Here's how the part is built. I have some questions about the finished solid (model axes, mm). Face numbers are marked on the shaded views. Coordinates: 2 decimals unless noted, no trailing zeros. Write each loop counter-clockwise with the first axis right and the second up, starting at its lowest first coordinate (ties: lowest second). Pieces come first, ordered by that corner, then holes. Notation, with made-up numbers: M -1,83 L 42,83 A6 cw 42,92 Z; hole C 5.25,23 d6. An arc over 180 degrees is marked long. Use a Markdown table: item, result.
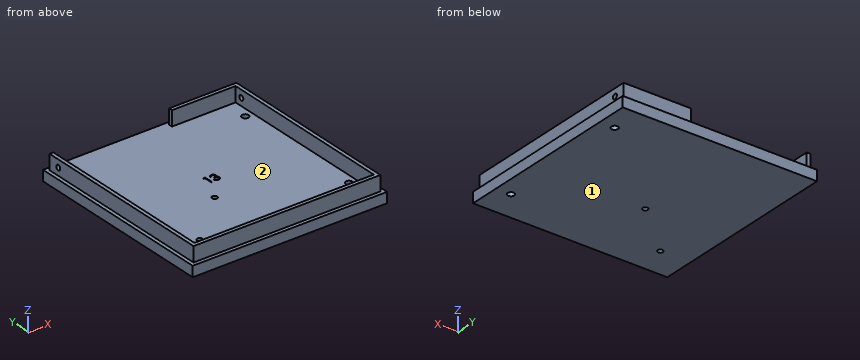
```python
from build123d import *

# Parameters (mm, degrees)
CROQUIS1_W              = 130
CROQUIS1_H              = 130
CROQUIS1_R              = 1.75
CROQUIS1_R_2            = 2.25
SALIENTE_EXTRUIR1_DEPTH = 7
CORTAR_EXTRUIR1_DEPTH   = 2
CROQUIS4_W              = 125
CROQUIS4_H              = 125
CROQUIS4_W_2            = 120
CROQUIS4_H_2            = 120
SALIENTE_EXTRUIR2_DEPTH = 10
CROQUIS6_R              = 1.7
CORTAR_EXTRUIR2_DEPTH   = 145.118874545
CORTAR_EXTRUIR3_REACH   = 146.119
CROQUIS7_W              = 77.5
CROQUIS7_H              = 10


with BuildPart() as part:
    # Croquis1 → Saliente-Extruir1 (new body)
    with BuildSketch(Plane.XY):
        Rectangle(CROQUIS1_W, CROQUIS1_H)
        with Locations((-11, -14)):
            Circle(CROQUIS1_R, mode=Mode.SUBTRACT)
        with Locations((-45, -45)):
            Circle(CROQUIS1_R, mode=Mode.SUBTRACT)
        with Locations((55, 45)):
            Circle(CROQUIS1_R_2, mode=Mode.SUBTRACT)
        with Locations((55, -45)):
            Circle(CROQUIS1_R_2, mode=Mode.SUBTRACT)
    extrude(amount=SALIENTE_EXTRUIR1_DEPTH)

    # Croquis2 → Cortar-Extruir1 (cut)
    with BuildSketch(Plane.XY.offset(7)):
        Polygon((-3.109375, 6), (-2, 6), (-2, 0), (-2.538461538, 0), (-2.538461538, 5.384615385), (-3.461538462, 5.384615385), align=None)
        with BuildLine():
            Line((1, 4.615384615), (0.461538462, 4.615384615))
            add(Edge.make_bspline(
                [(0.461538462, 4.615384615), (0.476126263, 4.675783159), (0.504644221, 4.793857373), (0.564125775, 4.962555534), (0.628924499, 5.122195856), (0.706734392, 5.269789126), (0.791606542, 5.40830153), (0.888845493, 5.534591458), (0.993965018, 5.651870827), (1.110236359, 5.755950663), (1.232171208, 5.850198199), (1.361487699, 5.93055544), (1.495584088, 5.999682559), (1.635389459, 6.056631528), (1.781320039, 6.099532426), (1.932056536, 6.130658378), (2.087993965, 6.150871717), (2.193846977, 6.152844454), (2.247596154, 6.153846154)],
                knots=[0, 0, 0, 0, 1.162005537, 2.271625781, 3.343758855, 4.383309926, 5.390229558, 6.379919256, 7.361854164, 8.333198761, 9.295911338, 10.242430842, 11.177959212, 12.116337295, 13.062827104, 14.020064771, 14.994644689, 16, 16, 16, 16], degree=3))
            add(Edge.make_bspline(
                [(2.247596154, 6.153846154), (2.325909426, 6.151481759), (2.48082773, 6.146804544), (2.708421525, 6.104094082), (2.927896072, 6.03650814), (3.136849069, 5.943124608), (3.33093781, 5.827946357), (3.503628416, 5.690863951), (3.652580149, 5.534522291), (3.777541939, 5.361837895), (3.875384795, 5.177285593), (3.947532863, 4.987342467), (3.991455745, 4.792459087), (3.997148128, 4.66087518), (4, 4.594951923)],
                knots=[0, 0, 0, 0, 1.083050992, 2.142477498, 3.193116406, 4.255571735, 5.30263384, 6.308962982, 7.297363603, 8.282367274, 9.249857812, 10.179914175, 11.08814088, 12, 12, 12, 12], degree=3))
            add(Edge.make_bspline(
                [(4, 4.594951923), (3.998005272, 4.531511704), (3.9941019, 4.407369039), (3.960958405, 4.226132187), (3.905181954, 4.055318015), (3.827919504, 3.894207451), (3.727905418, 3.743822011), (3.606752223, 3.603823341), (3.463604803, 3.473590499), (3.355126624, 3.398985688), (3.299278846, 3.360576923)],
                knots=[0, 0, 0, 0, 1.024540389, 2.004866551, 2.965041327, 3.920577974, 4.882998113, 5.874504559, 6.905732034, 8, 8, 8, 8], degree=3))
            add(Edge.make_bspline(
                [(3.299278846, 3.360576923), (3.363104711, 3.3297572), (3.48956221, 3.268694416), (3.661934546, 3.148941689), (3.818410904, 3.010673665), (3.905674422, 2.902771974), (3.949519231, 2.848557692)],
                knots=[0, 0, 0, 0, 1.015518401, 2.012035669, 3.001164323, 4, 4, 4, 4], degree=3))
            add(Edge.make_bspline(
                [(3.949519231, 2.848557692), (3.978390103, 2.809030118), (4.035659068, 2.730622261), (4.106348554, 2.604559817), (4.170478465, 2.477100121), (4.220450269, 2.344826853), (4.259148327, 2.209273116), (4.286810096, 2.070206151), (4.303994338, 1.927512398), (4.306455284, 1.830976718), (4.307692308, 1.782451923)],
                knots=[0, 0, 0, 0, 1.025084078, 2.033381695, 3.024893161, 4.013698104, 4.991890475, 5.976764909, 6.982997093, 8, 8, 8, 8], degree=3))
            add(Edge.make_bspline(
                [(4.307692308, 1.782451923), (4.304615999, 1.698435258), (4.298477858, 1.530797312), (4.243613731, 1.283126361), (4.158562461, 1.0410255), (4.037779142, 0.809468632), (3.890577699, 0.592816551), (3.715450857, 0.39897145), (3.514388443, 0.232345271), (3.290150187, 0.093127737), (3.047206539, -0.01816013), (2.787362667, -0.09540146), (2.514362574, -0.145708888), (2.327150064, -0.151103521), (2.231971154, -0.153846154)],
                knots=[0, 0, 0, 0, 0.955779014, 1.907060117, 2.875433937, 3.871313158, 4.872415639, 5.851225146, 6.836215519, 7.83643374, 8.849228613, 9.86973379, 10.916971861, 12, 12, 12, 12], degree=3))
            add(Edge.make_bspline(
                [(2.231971154, -0.153846154), (2.167823782, -0.152357788), (2.041603145, -0.149429181), (1.856042862, -0.129408722), (1.678919949, -0.092842999), (1.509994924, -0.043637332), (1.349117718, 0.018748511), (1.196779252, 0.096437708), (1.052042292, 0.187828854), (0.916272662, 0.294000719), (0.789486545, 0.41276873), (0.675053304, 0.546241319), (0.571065087, 0.691951154), (0.480306278, 0.851590679), (0.398642931, 1.023096834), (0.331475577, 1.208665688), (0.272357459, 1.406638298), (0.24487152, 1.544600138), (0.230769231, 1.615384615)],
                knots=[0, 0, 0, 0, 1.048658725, 2.063410685, 3.046034179, 4.001477787, 4.936774919, 5.862367409, 6.792675028, 7.730719943, 8.675894397, 9.627829632, 10.600096036, 11.597688215, 12.626045268, 13.701542398, 14.82072376, 16, 16, 16, 16], degree=3))
            Line((0.230769231, 1.615384615), (0.769230769, 1.615384615))
            add(Edge.make_bspline(
                [(0.769230769, 1.615384615), (0.783259269, 1.569186307), (0.810545919, 1.479326584), (0.856993287, 1.350000346), (0.909910325, 1.231443683), (0.96667814, 1.122786903), (1.026298333, 1.022959927), (1.093009633, 0.934602437), (1.161871025, 0.853833519), (1.213778488, 0.80832847), (1.239182692, 0.786057692)],
                knots=[0, 0, 0, 0, 1.198163088, 2.33053128, 3.407730985, 4.417276592, 5.372219308, 6.28897303, 7.162600585, 8, 8, 8, 8], degree=3))
            add(Edge.make_bspline(
                [(1.239182692, 0.786057692), (1.272776823, 0.760157691), (1.339861388, 0.708437637), (1.449178356, 0.642434845), (1.564146732, 0.585244516), (1.687257602, 0.54155818), (1.815854352, 0.504567905), (1.952015549, 0.480361301), (2.094539921, 0.463753007), (2.191856087, 0.46228741), (2.241586538, 0.461538462)],
                knots=[0, 0, 0, 0, 0.946170439, 1.889420265, 2.845303464, 3.807233317, 4.801018734, 5.828864929, 6.890507805, 8, 8, 8, 8], degree=3))
            add(Edge.make_bspline(
                [(2.241586538, 0.461538462), (2.2977354, 0.462594299), (2.407529652, 0.464658898), (2.567737982, 0.483645824), (2.72015075, 0.511297962), (2.863075765, 0.554005932), (2.998385206, 0.606773106), (3.12418232, 0.673027515), (3.242118502, 0.750761324), (3.350683197, 0.839114167), (3.448304067, 0.93583673), (3.534257518, 1.037001995), (3.607328367, 1.142183417), (3.666271643, 1.251963053), (3.712815444, 1.365886303), (3.744500931, 1.484272867), (3.766532099, 1.606153895), (3.768326292, 1.689003556), (3.769230769, 1.730769231)],
                knots=[0, 0, 0, 0, 1.217147791, 2.380027433, 3.494444702, 4.572153297, 5.609568379, 6.639424714, 7.649109417, 8.668170816, 9.669597737, 10.625200337, 11.543417969, 12.441394052, 13.322311151, 14.205496177, 15.095365482, 16, 16, 16, 16], degree=3))
            add(Edge.make_bspline(
                [(3.769230769, 1.730769231), (3.766607395, 1.786674383), (3.761373701, 1.898206512), (3.721416136, 2.062293782), (3.655692369, 2.22039106), (3.563682349, 2.369800986), (3.451678243, 2.50827396), (3.320766974, 2.631825073), (3.16986144, 2.7337738), (3.030970236, 2.804211497), (2.907944253, 2.852275055), (2.802660737, 2.884289279), (2.684792274, 2.911398403), (2.555764247, 2.93661944), (2.414604448, 2.958084609), (2.261466554, 2.975984864), (2.096319534, 2.990307791), (1.981991821, 2.996703955), (1.923076923, 3)],
                knots=[0, 0, 0, 0, 1.07054697, 2.135767047, 3.216561865, 4.33974944, 5.486079747, 6.621378074, 7.775625952, 8.963672916, 9.598146892, 10.304877434, 11.070270905, 11.915000392, 12.823868403, 13.805723172, 14.86925407, 16, 16, 16, 16], degree=3))
            Line((1.923076923, 3), (1.923076923, 3.615384615))
            add(Edge.make_bspline(
                [(1.923076923, 3.615384615), (1.997307493, 3.616644279), (2.142706944, 3.61911165), (2.355097181, 3.648953954), (2.558194287, 3.690235031), (2.747497274, 3.753466789), (2.920037925, 3.826907298), (3.069728672, 3.912368228), (3.194472353, 4.007364941), (3.293662761, 4.1133637), (3.368284296, 4.227046639), (3.42284452, 4.345532337), (3.455073651, 4.469859299), (3.459375937, 4.554707301), (3.461538462, 4.597355769)],
                knots=[0, 0, 0, 0, 1.321986639, 2.589447074, 3.816329219, 5.01088745, 6.139805852, 7.153945165, 8.075214402, 8.924034688, 9.728124013, 10.488707548, 11.240355623, 12, 12, 12, 12], degree=3))
            add(Edge.make_bspline(
                [(3.461538462, 4.597355769), (3.460828043, 4.628689047), (3.459414698, 4.691025116), (3.441590793, 4.782096662), (3.414806723, 4.870383998), (3.37798433, 4.955511673), (3.328698275, 5.036889285), (3.269716584, 5.115210626), (3.199485555, 5.190028533), (3.119007646, 5.259766224), (3.032587409, 5.326227773), (2.937873509, 5.382651151), (2.837721723, 5.430899829), (2.732021172, 5.470687547), (2.620428835, 5.500617755), (2.503469021, 5.522107769), (2.380918707, 5.535543748), (2.297310023, 5.537478176), (2.254807692, 5.538461538)],
                knots=[0, 0, 0, 0, 0.884392785, 1.759457502, 2.611959086, 3.489218968, 4.37281399, 5.2945488, 6.255912374, 7.266815255, 8.301784654, 9.332968512, 10.37626691, 11.440494194, 12.520033166, 13.637162961, 14.798855837, 16, 16, 16, 16], degree=3))
            add(Edge.make_bspline(
                [(2.254807692, 5.538461538), (2.186490547, 5.536076346), (2.053051273, 5.531417512), (1.860682844, 5.490612346), (1.6818497, 5.42550706), (1.545154843, 5.347793312), (1.444213288, 5.271078283), (1.372081394, 5.204079906), (1.301246233, 5.129623637), (1.23636793, 5.043123565), (1.170755398, 4.950437639), (1.111021864, 4.846854185), (1.052976678, 4.735075223), (1.018000878, 4.656054136), (1, 4.615384615)],
                knots=[0, 0, 0, 0, 1.472543308, 2.876219568, 4.221790263, 5.565193594, 6.249813518, 6.953379497, 7.687249741, 8.463570142, 9.283606569, 10.136032583, 11.040678096, 12, 12, 12, 12], degree=3))
        make_face()
    extrude(amount=-CORTAR_EXTRUIR1_DEPTH, mode=Mode.SUBTRACT)

    # Croquis4 → Saliente-Extruir2 (add)
    with BuildSketch(Plane.XY.offset(7)):
        Rectangle(CROQUIS4_W, CROQUIS4_H)
        Rectangle(CROQUIS4_W_2, CROQUIS4_H_2, mode=Mode.SUBTRACT)
    extrude(amount=SALIENTE_EXTRUIR2_DEPTH)

    # Croquis6 → Cortar-Extruir2 (cut, through all)
    with BuildSketch(Plane(origin=(62.5, 0, 0), x_dir=(0, 0, -1), z_dir=(1, 0, 0))):
        with Locations((-12, 55)):
            Circle(CROQUIS6_R)
    extrude(amount=-CORTAR_EXTRUIR2_DEPTH, mode=Mode.SUBTRACT)

    # Croquis7 → Cortar-Extruir3 (cut, up to next)
    with BuildSketch(Plane(origin=(0, 62.5, 0), x_dir=(1, 0, 0), z_dir=(0, 1, 0)), mode=Mode.PRIVATE) as cortar_extruir3_sk1:
        with Locations((-21.25, -12)):
            Rectangle(CROQUIS7_W, CROQUIS7_H)
    cortar_extruir3_tool1 = extrude(cortar_extruir3_sk1.sketch, amount=-CORTAR_EXTRUIR3_REACH, mode=Mode.PRIVATE) & part.part
    add(cortar_extruir3_tool1.solids().sort_by_distance((-21.25, 62.5, 12))[0], mode=Mode.SUBTRACT)


solid = part.part
```
1. Suppose I cut it at A-A on x = -45. Write out the boundary of the cut face in (y, z).
Answers follow:
| item | result |
|---|---|
| outline | M -65,0 L -46.75,0 L -46.75,7 L -60,7 L -60,17 L -62.5,17 L -62.5,7 L -65,7 Z; M -43.25,0 L 65,0 L 65,7 L -43.25,7 Z |
2. I need wall thicknesses on probe 1 along Y at (x, z) = (55, 2); probe 2 along Y at (x, z) = (37, 15); probe 3 along Y at (x, z) = (61.6, 12). Which ranges of each line are inside material? Lowest first, please.
Answers follow:
| item | result |
|---|---|
| probe 1 | y = -65 to -47.25, -42.75 to 42.75, 47.25 to 65 |
| probe 2 | y = -62.5 to -60, 60 to 62.5 |
| probe 3 | y = -62.5 to 53.3, 56.7 to 62.5 |
3. Suppose I cut it at C-C on x = 55. Write out the boundary of the cut face in (y, z), and give its area (3 significant figures).
Answers follow:
| item | result |
|---|---|
| outline | M -65,0 L -47.25,0 L -47.25,7 L -60,7 L -60,17 L -62.5,17 L -62.5,7 L -65,7 Z; M -42.75,0 L 42.75,0 L 42.75,7 L -42.75,7 Z; M 47.25,0 L 65,0 L 65,7 L 62.5,7 L 62.5,17 L 60,17 L 60,7 L 47.25,7 Z |
| area | 897 mm2 |
4. Suppose I cut it at D-D on y = -45. Write out the boundary of the cut face in (x, z), and give its area (3 significant figures).
Answers follow:
| item | result |
|---|---|
| outline | M -65,0 L -46.75,0 L -46.75,7 L -60,7 L -60,17 L -62.5,17 L -62.5,7 L -65,7 Z; M -43.25,0 L 52.75,0 L 52.75,7 L -43.25,7 Z; M 57.25,0 L 65,0 L 65,7 L 62.5,7 L 62.5,17 L 60,17 L 60,7 L 57.25,7 Z |
| area | 904 mm2 |
5. Suppose I cut it at B-B on y = 45. Write out the boundary of the cut face in (x, z), and give its area (4 significant figures).
Answers follow:
| item | result |
|---|---|
| outline | M -65,0 L 52.75,0 L 52.75,7 L -60,7 L -60,17 L -62.5,17 L -62.5,7 L -65,7 Z; M 57.25,0 L 65,0 L 65,7 L 62.5,7 L 62.5,17 L 60,17 L 60,7 L 57.25,7 Z |
| area | 928.5 mm2 |
6. Will these pins go through, and if not, where does the flat tip stop? pin 1 Ø3 at (x, y) = (-45, -45) entering from -Z; pin 2 Ø4.5 at (x, y) = (2, 2) entering from +Z; pin 3 Ø4 at (x, z) = (-33.5, 13) entering from -Y; pin 4 Ø5 at (x, z) = (-25, 10.5) entering from +Y.
Answers follow:
| item | result |
|---|---|
| pin 1 | passes through |
| pin 2 | stops at z = 7 |
| pin 3 | stops at y = -62.5 |
| pin 4 | stops at y = -60 |
7. We'd pull the mould along X, two halves only. Please class the marked faces 1 and 2: +X half, -X half, draft (parallel to the pull), parting line (faces both ways), or undercut.
Answers follow:
| item | result |
|---|---|
| face 1 | draft |
| face 2 | undercut |
